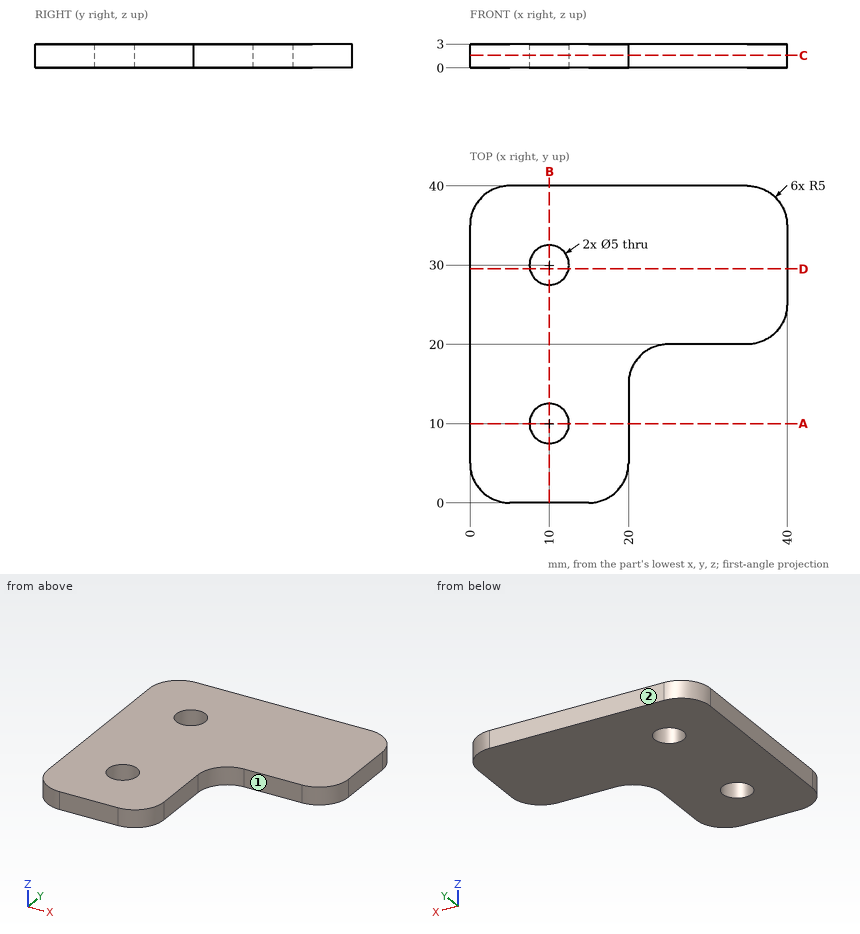
Geometry check sheet. Reference: drawing and pictorial views, mm from the part's lowest x, y, z. A direction names the side the tool comes from. Give positions to 0.01 mm unless a question says otherwise; leave off trailing zeros. Order: outer loops, then holes, each group sorted by start corner. A loop starts at its lowest first (then second) coordinate and runs counter-clockwise, first axis right, second up. Notation, with made-up numbers: M -9.5,26.5 L 33.5,26.5 A29 cw 33.5,59.5 Z; hole C 79,-34.75 d5. An arc over 180 degrees is marked long. Answer in a Markdown table with one row per item. Add a question column.
Q1. Gauge pin test, flat end, axial feed: pin 1 Ø1.5 at (y, z) = (8, 2) entering from +X. Record the tip position at first contact, or that the pin passes through.
Q2. Sectioned sample at D-D, the plane y = 29.5. Record the boundary of the cut face in (x, z).
Q3. Sectioned sample at C-C, the plane z = 1.55. Record the boundary of the cut face in (x, y).
Q4. Access from +Z, -Z, +X, -X, +Y, -Y to the whole of each face (thin tool, end or side, straight path). Record for the marked faces 1 and 2.
Q5. Sectioned sample at B-B, the plane x = 10. Record the boundary of the cut face in (y, z).
Q6. Sectioned sample at A-A, the plane y = 10. Record the boundary of the cut face in (x, z).
Q7. Thickness scan on L1, parallel to Y at x = 10, z = 0.7; L2, parallel to Y at x = 10.5, z = 1; L3, parallel to Y at x = 32.5, z = 0.6. Record the ranges inside material, lowest first.
Verdict:
| question | item | result |
|---|---|---|
| 1 | pin 1 | x = 20 |
| 2 | outline | M 0,0 L 7.55,0 L 7.55,3 L 0,3 Z; M 12.45,0 L 40,0 L 40,3 L 12.45,3 Z |
| 3 | outline | M 0,5 A5 ccw 5,0 L 15,0 A5 ccw 20,5 L 20,15 A5 cw 25,20 L 35,20 A5 ccw 40,25 L 40,35 A5 ccw 35,40 L 5,40 A5 ccw 0,35 Z; hole C 10,10 d5; hole C 10,30 d5 |
| 4 | face 1 | +Z, -Z, +X, -Y |
| 4 | face 2 | +Z, -Z, +X, -X, +Y |
| 5 | outline | M 0,0 L 7.5,0 L 7.5,3 L 0,3 Z; M 12.5,0 L 27.5,0 L 27.5,3 L 12.5,3 Z; M 32.5,0 L 40,0 L 40,3 L 32.5,3 Z |
| 6 | outline | M 0,0 L 7.5,0 L 7.5,3 L 0,3 Z; M 12.5,0 L 20,0 L 20,3 L 12.5,3 Z |
| 7 | L1 | 0 to 7.5, 12.5 to 27.5, 32.5 to 40 |
| 7 | L2 | 0 to 7.55, 12.45 to 27.55, 32.45 to 40 |
| 7 | L3 | 20 to 40 |
